Geometry check sheet. Reference: the model listing, model coordinates, mm. Round coordinates to 2 decimals unless told otherwise and drop trailing zeros. Order: outer loops, then holes, each group sorted by start corner. A loop starts at its lowest first (then second) coordinate and runs counter-clockwise, first axis right, second up.
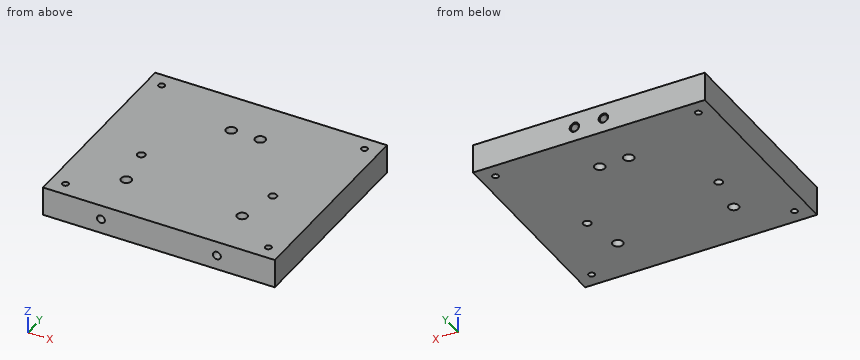
```python
from build123d import *

# Parameters (mm, degrees)
SKETCH1_W                       = 101.6
SKETCH1_H                       = 88.9
BOSS_EXTRUDE1_DEPTH             = 12.7
F_8_32_TAPPED_HOLE1_D           = 3.4544
F_8_32_TAPPED_HOLE1_DEPTH       = 19.05
F_8_32_TAPPED_HOLE1_CSINK_D     = 4.1656
F_8_32_TAPPED_HOLE1_CSINK_ANGLE = 90
F_8_32_TAPPED_HOLE1_TIP         = 1.037806461
F_8_CLEARANCE_HOLE2_D           = 4.4958
F_8_CLEARANCE_HOLE2_DEPTH       = 25.4
F_8_CLEARANCE_HOLE2_TIP         = 1.350674586
F_6_32_TAPPED_HOLE1_D           = 2.7051
F_8_32_TAPPED_HOLE2_D           = 3.4544
F_8_32_TAPPED_HOLE3_D           = 3.4544
F_8_32_TAPPED_HOLE3_DEPTH       = 19.05
F_8_32_TAPPED_HOLE3_TIP         = 1.037806461
F_8_CLEARANCE_HOLE3_D           = 4.4958
F_8_CLEARANCE_HOLE3_DEPTH       = 19.05
F_8_CLEARANCE_HOLE3_TIP         = 1.350674586


with BuildPart() as part:
    # Sketch1 → Boss-Extrude1 (new body)
    with BuildSketch(Plane.XY):
        with Locations((-50.8, 44.45)):
            Rectangle(SKETCH1_W, SKETCH1_H)
    extrude(amount=BOSS_EXTRUDE1_DEPTH)

    # #8-32 Tapped Hole1
    with Locations(Plane(origin=(0, 88.9, 0), x_dir=(1, 0, 0), z_dir=(0, 1, 0))):
        with Locations((-44.45, -6.35), (-57.15, -6.35)):
            CounterSinkHole(F_8_32_TAPPED_HOLE1_D / 2, F_8_32_TAPPED_HOLE1_CSINK_D / 2, depth=F_8_32_TAPPED_HOLE1_DEPTH, counter_sink_angle=F_8_32_TAPPED_HOLE1_CSINK_ANGLE)
            with Locations((0, 0, -(F_8_32_TAPPED_HOLE1_DEPTH + F_8_32_TAPPED_HOLE1_TIP / 2))):  # 118° drill point
                Cone(0, F_8_32_TAPPED_HOLE1_D / 2, F_8_32_TAPPED_HOLE1_TIP, mode=Mode.SUBTRACT)

    # #8 Clearance Hole2
    with Locations(Plane.XY.offset(12.7)):
        with Locations((-44.45, 68.812193539), (-57.15, 68.812193539)):
            Hole(F_8_CLEARANCE_HOLE2_D / 2, depth=F_8_CLEARANCE_HOLE2_DEPTH)
            with Locations((0, 0, -(F_8_CLEARANCE_HOLE2_DEPTH + F_8_CLEARANCE_HOLE2_TIP / 2))):  # 118° drill point
                Cone(0, F_8_CLEARANCE_HOLE2_D / 2, F_8_CLEARANCE_HOLE2_TIP, mode=Mode.SUBTRACT)

    # #6-32 Tapped Hole1 (through all)
    with Locations(Plane.XY.offset(12.7)):
        with Locations((-95.25, 6.35), (-95.25, 82.55), (-6.35, 6.35), (-6.35, 82.55)):
            Hole(F_6_32_TAPPED_HOLE1_D / 2)

    # #8-32 Tapped Hole2 (through all)
    with Locations(Plane(origin=(0, 0, 0), x_dir=(-1, 0, 0), z_dir=(0, 0, -1))):
        with Locations((79.3203, 37.592), (21.675, 37.592)):
            Hole(F_8_32_TAPPED_HOLE2_D / 2)

    # #8-32 Tapped Hole3
    with Locations(Plane(origin=(0, 0, 0), x_dir=(-1, 0, 0), z_dir=(0, -1, 0))):
        with Locations((76.2, -6.35), (25.4, -6.35)):
            Hole(F_8_32_TAPPED_HOLE3_D / 2, depth=F_8_32_TAPPED_HOLE3_DEPTH)
            with Locations((0, 0, -(F_8_32_TAPPED_HOLE3_DEPTH + F_8_32_TAPPED_HOLE3_TIP / 2))):  # 118° drill point
                Cone(0, F_8_32_TAPPED_HOLE3_D / 2, F_8_32_TAPPED_HOLE3_TIP, mode=Mode.SUBTRACT)

    # #8 Clearance Hole3
    with Locations(Plane.XY.offset(12.7)):
        with Locations((-76.2, 20.087806461), (-25.4, 20.087806461)):
            Hole(F_8_CLEARANCE_HOLE3_D / 2, depth=F_8_CLEARANCE_HOLE3_DEPTH)
            with Locations((0, 0, -(F_8_CLEARANCE_HOLE3_DEPTH + F_8_CLEARANCE_HOLE3_TIP / 2))):  # 118° drill point
                Cone(0, F_8_CLEARANCE_HOLE3_D / 2, F_8_CLEARANCE_HOLE3_TIP, mode=Mode.SUBTRACT)


solid = part.part
```
(1) Sectioned sample at C-C, the plane x = -25.4. Record the cut outline in (y, z), and give its area (3 significant figures).
Returned:
outline: (0, 0) - (17.84, 0) - (17.84, 4.62) - (0, 4.62) - close; (0, 8.08) - (17.84, 8.08) - (17.84, 12.7) - (0, 12.7) - close; (22.34, 0) - (88.9, 0) - (88.9, 12.7) - (22.34, 12.7) - close
area: 1,010 mm2
(2) Depth check by flat-ended pin: P1, Ø4, axis at x = -83.5, z = 7.5, coming from the -Y side; P2, Ø1.6, axis at x = -6.35, y = 82.55, coming from the -Z side; P3, Ø2, axis at x = -76.2, z = 6.35, coming from the -Y side; P4, Ø3, axis at x = -44.45, z = 6.35, coming from the +Y side. Enter the tip coordinate at first touch or a pass-through.
Returned:
P1: stops at y = 0
P2: passes through
P3: stops at y = 22.1
P4: stops at y = 67.14
(3) Sectioned sample at A-A, the plane y = 6.35. Record the cut outline in (x, z), and give its area (3 significant figures).
Returned:
outline: (-101.6, 0) - (-96.6, 0) - (-96.6, 12.7) - (-101.6, 12.7) - close; (-93.9, 0) - (-7.7, 0) - (-7.7, 12.7) - (-93.9, 12.7) - close; (-5, 0) - (0, 0) - (0, 12.7) - (-5, 12.7) - close; hole circle Ø3.45 at (-76.2, 6.35); hole circle Ø3.45 at (-25.4, 6.35)
area: 1,200 mm2
(4) Sectioned sample at B-B, the plane x = -44.45. Record the cut outline in (y, z).
Returned:
outline: (0, 0) - (66.56, 0) - (66.56, 12.7) - (0, 12.7) - close; (71.06, 0) - (88.9, 0) - (88.9, 4.27) - (88.54, 4.62) - (71.06, 4.62) - close; (71.06, 8.08) - (88.54, 8.08) - (88.9, 8.43) - (88.9, 12.7) - (71.06, 12.7) - close
(5) Material ranges on line 1 (X direction, y = 13.25, z = 6.35); line 2 (Y direction, x = -6.35, z = 7.25); line 3 (X direction, y = 76.5, z = 6.35), recorded low to high.
Returned:
line 1: x = -101.6 to -77.93, -74.47 to -27.13, -23.67 to 0
line 2: y = 0 to 5, 7.7 to 81.2, 83.9 to 88.9
line 3: x = -101.6 to -58.88, -55.42 to -46.18, -42.72 to 0
(6) Sectioned sample at D-D, the plane x = -95.25. Record the cut outline in (y, z), and give its area (3 significant figures).
Returned:
outline: (0, 0) - (5, 0) - (5, 12.7) - (0, 12.7) - close; (7.7, 0) - (81.2, 0) - (81.2, 12.7) - (7.7, 12.7) - close; (83.9, 0) - (88.9, 0) - (88.9, 12.7) - (83.9, 12.7) - close
area: 1,060 mm2
